Here's how the part is built. I have some questions about the finished solid (model axes, mm). Face numbers are marked on the shaded views. A direction names the side the tool comes from. Coordinates: 2 decimals unless noted, no trailing zeros. Loops run counter-clockwise (first coordinate to the right, second up) from the corner with the lowest first, then second, coordinate; pieces in that order, holes last. Notation, with made-up numbers: M 54.5,28.5 L 66.5,28.5 A28 cw 66.5,53.5 Z; hole C 65.25,-1.75 d9. An arc over 180 degrees is marked long. Use one line per item in the form item = value. Start each with the question number.
(1) Please list where these lines run through material, in increasing order: L1, parallel to Y at x = -20, z = -1; L2, parallel to Z at x = -43, y = 19; L3, parallel to Z at x = 36, y = 18.
(2) On a 3-axis mill with a long thin cutter (end or side, diameter ignored), from which of +Z, -Z, +X, -X, +Y, -Y can I reach the whole of each face in a straight line? I mean the marked faces 5 and 6. Say none if no direction works.
(3) Thinking about a two-plate mould opening in X: for the marked faces 1, 2, 3 and 4, which applies, +X half, -X half, draft (parallel to the pull), parting line (faces both ways), or undercut?
(4) Imagine slicing it at B-B, the plane x = -33. Please give me the cut outline in (y, z).
(5) Imagine slicing it at A-A, the plane x = -45.5. Please give me the cut outline in (y, z).
(6) Will these pins go through, and if not, where does the flat tip stop? P1, Ø1, axis at x = 36, z = 33.5, coming from the -Y side; P2, Ø2, axis at x = -24, z = -10.5, coming from the -Y side; P3, Ø3, axis at y = 0, z = -7.5, coming from the +X side.
```python
from build123d import *

# Parameters (mm, degrees)
R_VOLUTION3_OUTLINE_W = 12
R_VOLUTION3_OUTLINE_H = 12
ESQUISSE2_R           = 21.001288109
ESQUISSE2_R_2         = 9
BOSS_EXTRU_1_DEPTH    = 80
ESQUISSE3_R           = 11.037807833
BOSS_EXTRU_2_DEPTH    = 5
CONG_1_R              = 4


# Read off the part's stored shape, not the designer's step: Révolution3
with BuildPart() as part:
    # Révolution3 outline → Révolution3 (revolve)
    with BuildSketch(Plane.YX):
        with BuildLine():
            add(Edge.make_bspline(
                [(9, 0), (9.053826316, 3.507535605), (9.211693628, 27.185630898), (15.14970787, 42)],
                knots=[0, 0, 0, 0, 0.679566397, 0.679566397, 0.679566397, 0.679566397], degree=3))
            Line((9, 0), (21.001288109, 0))
            Line((21.001288109, 0), (21.001288109, 42))
            Line((21.001288109, 42), (15.14970787, 42))
        make_face()
        with BuildLine():
            add(Edge.make_bspline(
                [(15.14970787, 42), (16.682530626, 45.824140722), (18.600512592, 49.057648401), (21.001288109, 51.201106105)],
                knots=[0.679566397, 0.679566397, 0.679566397, 0.679566397, 0.854987808, 0.854987808, 0.854987808, 0.854987808], degree=3))
            Line((15.14970787, 42), (21.001288109, 42))
            Line((21.001288109, 42), (21.001288109, 51.201106105))
        make_face()
        with BuildLine():
            Line((21.001288109, 42), (21.001288109, 0))
            add(Edge.make_bspline(
                [(28, 42), (27.997779305, 41.997025444), (27.875050115, 41.83237842), (27.609034397, 41.447212382), (27.160528215, 40.690969165), (26.526197616, 39.457776411), (25.708310332, 37.527019057), (24.777928166, 34.714134126), (23.942034299, 31.528478566), (22.978703398, 26.934375104), (22.072778857, 20.805167001), (21.526924747, 14.790080699), (21.257611914, 10.390059795), (21.125442102, 7.378245527), (21.048712817, 4.734783543), (21.018586389, 2.904179393), (21.007225123, 1.69657239), (21.003198587, 0.929954604), (21.001909089, 0.369945076), (21.0015083, 0.102272875), (21.001288109, 0)],
                knots=[0.198795247, 0.198795247, 0.198795247, 0.198795247, 0.199272098, 0.22510203, 0.250931963, 0.276761895, 0.32842176, 0.380081624, 0.431741489, 0.483401354, 0.586721083, 0.690040812, 0.741700677, 0.793360541, 0.845020406, 0.896680271, 0.922510203, 0.948340135, 0.974170068, 0.990325422, 0.990325422, 0.990325422, 0.990325422], degree=3))
            Line((28, 42), (21.001288109, 42))
        make_face()
        with BuildLine():
            add(Edge.make_bspline(
                [(21.001288109, 51.201106105), (22.985890317, 52.972996421), (25.300409981, 54), (28, 54)],
                knots=[0.854987808, 0.854987808, 0.854987808, 0.854987808, 1, 1, 1, 1], degree=3))
            Line((21.001288109, 51.201106105), (21.001288109, 42))
            Line((21.001288109, 42), (28, 42))
            Line((28, 42), (28, 54))
        make_face()
        Polygon((40, 42), (28, 42), (28, 0), (40, 0), (40, 31.2), align=None)
        with Locations((34, 48)):
            Rectangle(R_VOLUTION3_OUTLINE_W, R_VOLUTION3_OUTLINE_H)
        Polygon((40, 0), (28, 0), (28, -54), (40, -54), (40, -31.2), align=None)
        with BuildLine():
            Line((50.8, 42), (40, 42))
            Line((40, 42), (40, 31.2))
            ThreePointArc((40, 31.2), (43.163246763, 38.836753237), (50.8, 42))
        make_face()
        Polygon((40, 54), (40, 42), (50.8, 42), (52, 42), (52, 54), align=None)
        with BuildLine():
            Line((40, -31.2), (40, -54))
            Line((40, -54), (52, -54))
            Line((52, -54), (52, -42))
            Line((52, -42), (50.8, -42))
            ThreePointArc((50.8, -42), (43.163246763, -38.836753237), (40, -31.2))
        make_face()
    revolve(axis=Axis((0, 0, 0), (1, 0, 0)))

    # Esquisse2 → Boss.-Extru.1 (add)
    with BuildSketch(Plane.ZY.offset(54)):
        Circle(ESQUISSE2_R)
        Circle(ESQUISSE2_R_2, mode=Mode.SUBTRACT)
    extrude(amount=-BOSS_EXTRU_1_DEPTH)

    # Esquisse3 → Boss.-Extru.2 (add)
    with BuildSketch(Plane(origin=(26, 0, 0), x_dir=(0, 0, -1), z_dir=(1, 0, 0))):
        with Locations(Location((0, 0, 0), (0, 0, 180))):
            Circle(ESQUISSE3_R)
    extrude(amount=BOSS_EXTRU_2_DEPTH)

    # Congé1
    cong_1_edges = [part.edges().sort_by_distance(p)[0] for p in [
        (31, 0, -11.037807833),
    ]]
    fillet(cong_1_edges, radius=CONG_1_R)


solid = part.part
```
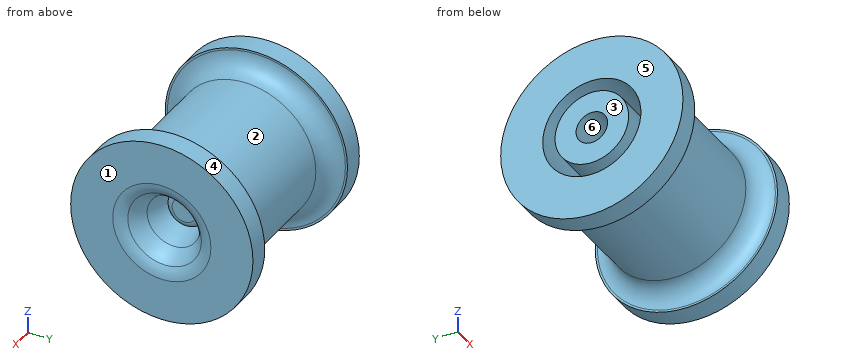
Answer:
q1.L1 = -39.99 to -27.98, -20.98 to -8.94, 8.94 to 20.98, 27.98 to 39.99
q1.L2 = -48.4 to -20.57, -8.95 to 8.95, 20.57 to 48.4
q1.L3 = -36.98 to -21.45, -17.65 to 17.65, 21.45 to 36.98
q2.face_5 = +Z, -Z, -X, +Y, -Y
q2.face_6 = -X
q3.face_1 = +X half
q3.face_2 = undercut
q3.face_3 = -X half
q3.face_4 = draft
q4.outline = C 0,0 d80.3; C 0,0 d42; hole C 0,0 d56; hole C 0,0 d18
q5.outline = C 0,0 d104; C 0,0 d42; hole C 0,0 d56; hole C 0,0 d18
q6.P1 = -24.67
q6.P2 = -38.86
q6.P3 = 31
